Part model, mm, in its own coordinate system. A direction names the side the tool comes from. Give positions to 0.01 mm unless a question says otherwise; leave off trailing zeros. Loops run counter-clockwise (first coordinate to the right, second up) from the corner with the lowest first, then second, coordinate; pieces in that order, holes last. Notation, with made-up numbers: M 45.25,20 L 90.25,20 A17 ccw 90.25,28 Z; hole C 59.5,87.5 d6. An arc over 180 degrees is marked long. Answer in a Markdown table with one row per item.
from build123d import *

# Parameters (mm, degrees)
SKETCH1_W                            = 70.5
SKETCH1_H                            = 101.8
SKETCH1_W_2                          = 66.5
SKETCH1_H_2                          = 97.8
BOSS_EXTRUDE1_BOARD_4MM_DEPTH        = 10
SKETCH2_W                            = 101.8
SKETCH2_H                            = 70.5
BOSS_EXTRUDE2_UNDER_10MS_DEPTH       = 10
SKETCH3_W                            = 101.8
SKETCH3_H                            = 70.5
BOSS_EXTRUDE3_BOTTOM_COVER_2MM_DEPTH = 2
SKETCH4_W                            = 5
SKETCH4_H                            = 3.5
BOSS_EXTRUDE4_DEPTH                  = 2
SKETCH5_W                            = 128.386338002
SKETCH5_H                            = 40
CUT_EXTRUDE1_CUT_USB_DEPTH           = 15
CUT_EXTRUDE1_CUT_USB_DRAFT           = -20
FILLET1_R                            = 2
CHAMFER2_START                       = 2.1
CHAMFER2_DEPTH                       = 2
CHAMFER2_2_DEPTH                     = 2


with BuildPart() as part:
    # Sketch1 → Boss-Extrude1-board-4mm (new body)
    with BuildSketch(Plane(origin=(0, 0, 0), x_dir=(0, 1, 0), z_dir=(0, 0, 1))):
        Rectangle(SKETCH1_W, SKETCH1_H)
        Rectangle(SKETCH1_W_2, SKETCH1_H_2, mode=Mode.SUBTRACT)
    extrude(amount=BOSS_EXTRUDE1_BOARD_4MM_DEPTH)

    # Sketch2 → Boss-Extrude2-under-10ms (add)
    with BuildSketch(Plane(origin=(0, 0, 0), x_dir=(1, 0, 0), z_dir=(0, 0, -1))):
        Rectangle(SKETCH2_W, SKETCH2_H)
        Polygon((-48.9, 30.25), (-38.9, 30.25), (-38.9, 33.25), (38.9, 33.25), (38.9, 30.25), (48.9, 30.25), (48.9, -30.25), (38.9, -30.25), (38.9, -33.25), (-38.9, -33.25), (-38.9, -30.25), (-48.9, -30.25), align=None, mode=Mode.SUBTRACT)
    extrude(amount=BOSS_EXTRUDE2_UNDER_10MS_DEPTH)

    # Sketch3 → Boss-Extrude3-bottom-cover-2mm (add)
    with BuildSketch(Plane(origin=(0, 0, -10), x_dir=(1, 0, 0), z_dir=(0, 0, -1))):
        Rectangle(SKETCH3_W, SKETCH3_H)
    extrude(amount=BOSS_EXTRUDE3_BOTTOM_COVER_2MM_DEPTH)

    # Sketch4 → Boss-Extrude4 (add)
    with BuildSketch(Plane.XY.offset(2.1)):
        with Locations((-16.4, 33.5)):
            Rectangle(SKETCH4_W, SKETCH4_H)
        with Locations((-16.4, -33.5)):
            Rectangle(SKETCH4_W, SKETCH4_H)
        with Locations((16.4, -33.5)):
            Rectangle(SKETCH4_W, SKETCH4_H)
        with Locations((16.4, 33.5)):
            Rectangle(SKETCH4_W, SKETCH4_H)
    extrude(amount=BOSS_EXTRUDE4_DEPTH)


with BuildPart() as cut_extrude1_cut_usb_tool:
    # Sketch5 → Cut-Extrude1-cut-usb (with draft: the straight prism first)
    with BuildSketch(Plane.XY.offset(10)):
        Rectangle(SKETCH5_W, SKETCH5_H)
    extrude(amount=-CUT_EXTRUDE1_CUT_USB_DEPTH)
    # Cut-Extrude1-cut-usb: the draft: its side faces are tilted about the plane it starts from
    cut_extrude1_cut_usb_sides = [cut_extrude1_cut_usb_tool.faces().sort_by_distance(p)[0] for p in [
        (0, -20, 2.5),
        (64.193169001, 0, 2.5),
        (0, 20, 2.5),
        (-64.193169001, 0, 2.5),
    ]]
    draft(cut_extrude1_cut_usb_sides, Plane.XY.offset(10), CUT_EXTRUDE1_CUT_USB_DRAFT)


with BuildPart() as part_1:
    add(part.part)

    # Cut-Extrude1-cut-usb: cut by cut_extrude1_cut_usb_tool
    add(cut_extrude1_cut_usb_tool.part, mode=Mode.SUBTRACT)

    # Fillet1
    fillet1_edges = [part_1.edges().sort_by_distance(p)[0] for p in [
        (50.9, -35.25, -1),
        (-50.9, -35.25, -1),
        (-50.9, 35.25, -1),
        (50.9, 35.25, -1),
    ]]
    fillet(fillet1_edges, radius=FILLET1_R)

    # Chamfer2: read off the stored shape, not the designer's step
    # Chamfer2 outline → Chamfer2 (cut)
    with BuildSketch(Plane.XY.offset(CHAMFER2_START)):
        Polygon((-18.9, -31.75), (-18.9, -33.25), (-17.4, -31.75), align=None)
        Polygon((-13.9, -31.75), (-15.4, -31.75), (-13.9, -33.25), align=None)
        Polygon((13.9, -31.75), (13.9, -33.25), (15.4, -31.75), align=None)
        Polygon((18.9, -31.75), (17.4, -31.75), (18.9, -33.25), align=None)
    extrude(amount=CHAMFER2_DEPTH, mode=Mode.SUBTRACT)

    # Chamfer2 2 outline → Chamfer2 2 (add)
    with BuildSketch(Plane.XY.offset(CHAMFER2_START)):
        Polygon((-18.9, 31.75), (-18.9, 33.25), (-20.4, 33.25), align=None)
        Polygon((-13.9, 31.75), (-12.4, 33.25), (-13.9, 33.25), align=None)
        Polygon((20.4, 33.25), (18.9, 33.25), (18.9, 31.75), align=None)
        Polygon((12.4, 33.25), (13.9, 31.75), (13.9, 33.25), align=None)
    extrude(amount=CHAMFER2_2_DEPTH)


solid = part_1.part
(1) Pull direction X, two halves, no side cores. Call faces 1 (the face through (44, -30.25, -5)), 2 (the face through (49.89, 17.31, 2.61)), 3 (the face through (50.9, 0, -6)): +X half, -X half, draft (parallel to the pull), parting line (faces both ways), or undercut.
Recorded:
| item | result |
|---|---|
| face 1 | undercut |
| face 2 | draft |
| face 3 | +X half |
(2) Drill centre lines: line 1 along X through (y, z) = (-22.5, 5.25); line 2 along Y through (x, z) = (-26.5, -0.5); line 3 along Z through (x, y) = (3, -28). Where is each one in solid material? Low to high.
Recorded:
| item | result |
|---|---|
| line 1 | x = -50.9 to -48.9, 48.9 to 50.9 |
| line 2 | y = -35.25 to -33.25, 33.25 to 35.25 |
| line 3 | z = -12 to -10 |
(3) Saw through at D-D (x = -44). Write the cut outline in (y, z).
Recorded:
| item | result |
|---|---|
| outline | M -35.25,-12 L 35.25,-12 L 35.25,10 L 33.25,10 L 33.25,0 L 30.25,0 L 30.25,-10 L -30.25,-10 L -30.25,0 L -33.25,0 L -33.25,10 L -35.25,10 Z |
(4) Saw through at B-B (y = 3). Write the cut outline in (x, z).
Recorded:
| item | result |
|---|---|
| outline | M -50.9,-12 L 50.9,-12 L 50.9,-5 L 48.9,-5 L 48.9,-10 L -48.9,-10 L -48.9,-5 L -50.9,-5 Z |
(5) Which spindle directions (+Z, -Z, +X, -X, +Y, -Y) get a long thin tool onto all of the face, cutting with end or side? Do faces 4 (the face through (49.886, -17.308, 2.605)), 5 (the face through (-38.9, -32, -5)), 6 (the face through (-50.33, -34.65, -0.85)). Say none if no direction does.
Recorded:
| item | result |
|---|---|
| face 4 | +Z, +X, -X |
| face 5 | +Z |
| face 6 | +Z, -Z, -X, -Y |
(6) Pin check, flat tips, straight feed: pin 1 Ø6 at (x, y) = (-4, 5.5) entering from +Z; pin 2 Ø2.5 at (x, y) = (46, 32.5) entering from +Z. Stop position of each tip, or through.
Recorded:
| item | result |
|---|---|
| pin 1 | stops at z = -10 |
| pin 2 | stops at z = 10 |
(7) Saw through at C-C (z = 5.75). Write the cut outline in (x, y).
Recorded:
| item | result |
|---|---|
| outline | M -50.9,-33.25 A2 ccw -48.9,-35.25 L 48.9,-35.25 A2 ccw 50.9,-33.25 L 50.9,-18.45 L 48.9,-18.45 L 48.9,-33.25 L -48.9,-33.25 L -48.9,-18.45 L -50.9,-18.45 Z; M -50.9,18.45 L -48.9,18.45 L -48.9,33.25 L 48.9,33.25 L 48.9,18.45 L 50.9,18.45 L 50.9,33.25 A2 ccw 48.9,35.25 L -48.9,35.25 A2 ccw -50.9,33.25 Z |
(8) Saw through at A-A (z = -8.5). Write the cut outline in (x, y), plus the area to 3 significant figures.
Recorded:
| item | result |
|---|---|
| outline | M -50.9,-33.25 A2 ccw -48.9,-35.25 L 48.9,-35.25 A2 ccw 50.9,-33.25 L 50.9,33.25 A2 ccw 48.9,35.25 L -48.9,35.25 A2 ccw -50.9,33.25 Z; hole M -48.9,-30.25 L -38.9,-30.25 L -38.9,-33.25 L 38.9,-33.25 L 38.9,-30.25 L 48.9,-30.25 L 48.9,30.25 L 38.9,30.25 L 38.9,33.25 L -38.9,33.25 L -38.9,30.25 L -48.9,30.25 Z |
| area | 790 mm^2 |
